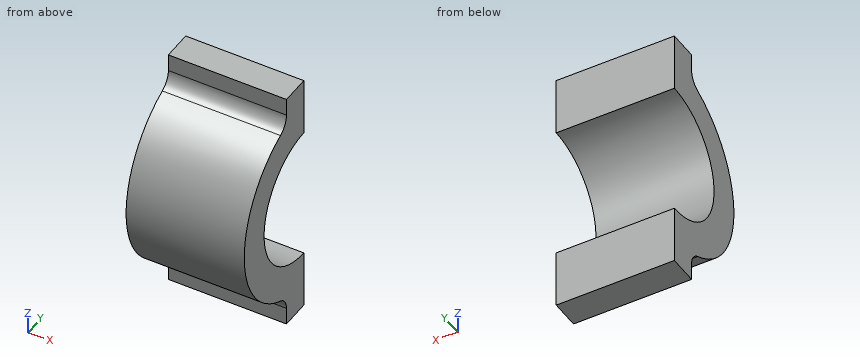
```python
from build123d import *

# Parameters (mm, degrees)
F1_DEPTH = 35
F2_R     = 5


with BuildPart() as f1:
    # F0 (on Right) → F1 (new body)
    with BuildSketch(Plane.YZ):
        with BuildLine():
            ThreePointArc((0, -20), (-20, 0), (0, 20))
            Line((0, 20), (0, 37.416574))
            Line((0, 37.416574), (-8.708287, 37.416574))
            Line((-8.708287, 37.416574), (-8.708287, 28.708287))
            ThreePointArc((-8.708287, 28.708287), (-30, 0), (-8.708287, -28.708287))
            Line((-8.708287, -28.708287), (-8.708287, -37.416574))
            Line((-8.708287, -37.416574), (0, -37.416574))
            Line((0, -37.416574), (0, -20))
        make_face()
    extrude(amount=F1_DEPTH)

    # F2
    f2_edges = [f1.edges().sort_by_distance(p)[0] for p in [
        (17.5, -8.708287, 28.708287),
        (17.5, -8.708287, -28.708287),
    ]]
    fillet(f2_edges, radius=F2_R)


solid = f1.part
```
Design review of the part built by this model. Coordinates are the model's own, in mm. Coordinates: 2 decimals unless noted, no trailing zeros. Order: outer loops, then holes, each group sorted by start corner. A loop starts at its lowest first (then second) coordinate and runs counter-clockwise, first axis right, second up.
1) Wall thickness on line 1 along Z through (x, y) = (28, -10); line 2 along Z through (x, y) = (29.5, -7.5); line 3 along Y through (x, z) = (32, -32): over which ranges is each line inside the solid? List them lowest first.
2) Clearance check with flat-ended pins moving along their axes: pin 1 (5.5 mm diameter, centred on x = 19.5, z = -34, fed in from -Y); pin 2 (3 mm diameter, centred on x = 19.5, z = 10, fed in from -Y); pin 3 (1.5 mm diameter, centred on x = 10.5, y = -19, fed in from +Z). State where each tip first meets the part, or that it passes through.
3) Take a section at D-D, the plane y = -24. Give the boundary of the cut face in (x, z), and give its area (3 significant figures).
4) Take a section at C-C, the plane z = 3.5. Give the boundary of the cut face in (x, y).
5) Take a section at B-B, the plane y = -15. Give the boundary of the cut face in (x, z).
6) Take a section at A-A, the plane x = 16. Give the boundary of the cut face in (y, z).
Returned:
1. line 1: z = -28.85 to -17.32, 17.32 to 28.85
1. line 2: z = -37.42 to -18.54, 18.54 to 37.42
1. line 3: y = -8.71 to 0
2. pin 1: stops at y = -8.8
2. pin 2: stops at y = -28.77
2. pin 3: stops at z = 23.81
3. outline: (0, -18) - (35, -18) - (35, 18) - (0, 18) - close
3. area: 1,260 mm2
4. outline: (0, -29.8) - (35, -29.8) - (35, -19.69) - (0, -19.69) - close
5. outline: (0, -25.98) - (35, -25.98) - (35, -13.23) - (0, -13.23) - close; (0, 13.23) - (35, 13.23) - (35, 25.98) - (0, 25.98) - close
6. outline: (-11.75, -27.6) arc R5 cw to (-8.71, -32.2) - (-8.71, -37.42) - (0, -37.42) - (0, -20) arc R20 cw to (0, 20) - (0, 37.42) - (-8.71, 37.42) - (-8.71, 32.2) arc R5 cw to (-11.75, 27.6) arc R30 ccw to start
